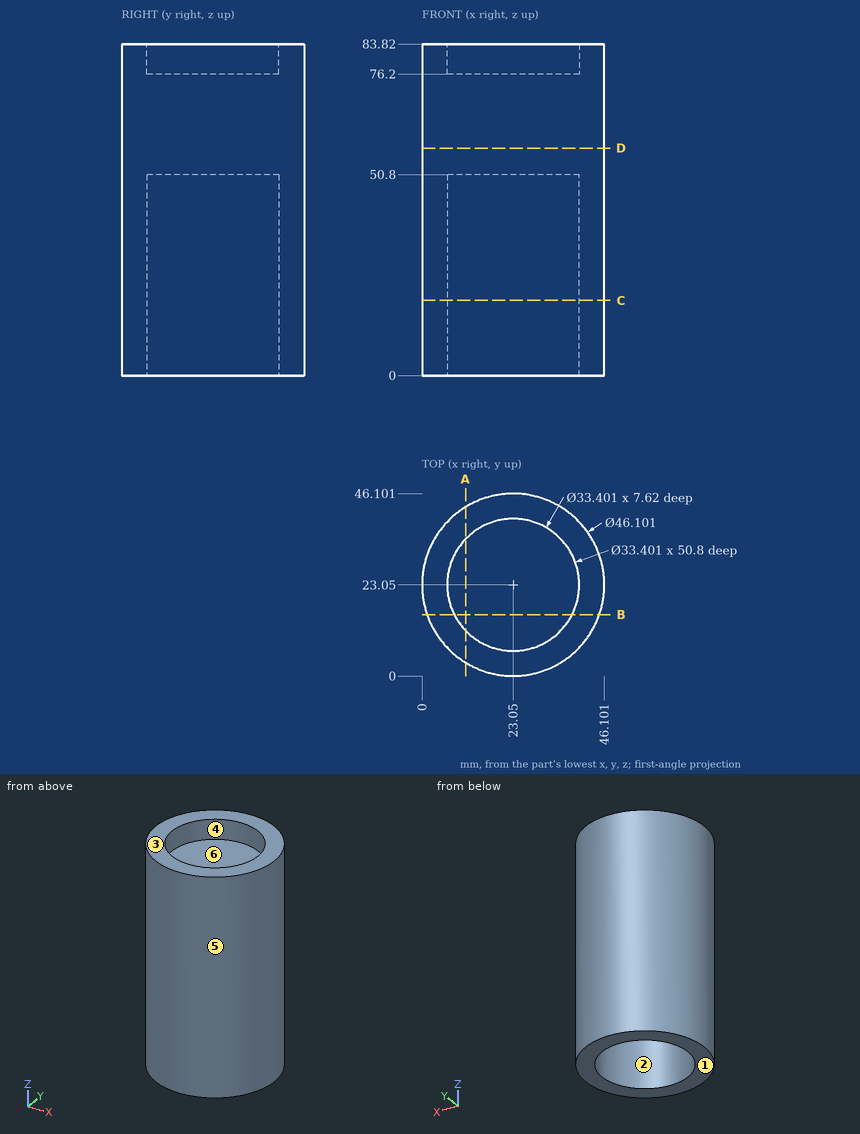
Answer from the drawing. Dimensions are ordinates in mm from the lowest x, y and z of the part. A direction names the side the tool comes from. Coordinates: 2 decimals unless noted, no trailing zeros. Write each loop counter-clockwise with the first axis right and the second up, starting at its lowest first coordinate (ties: lowest second). Pieces come first, ordered by that corner, then holes. Notation, with made-up numbers: M 42,42.25 L 48,42.25 A12 cw 48,62.25 Z; hole C 85.5,22.5 d3. An arc over 180 degrees is marked long. Use one line per item in the form item = value. Start each with the question number.
1. The part is cut by section A-A (x = 11). Give the vertices of the cut face in (y, z), plus the area to 3 significant figures.
2. Straight lines are drawn through the part: probe 1 along Z at (x, y) = (37, 22); probe 2 along Y at (x, z) = (18, 78); probe 3 along X at (y, z) = (15, 22.5). For each, find the intervals that lie inside material, in ascending order. Write a range as from..to.
3. The part is cut by section C-C (z = 19). Give the vertices of the cut face in (x, y).
4. A tool of negligible diameter and unlimited length cuts with its end or side. For the marked faces 1 and 2, from which of +Z, -Z, +X, -X, +Y, -Y can it reach the whole face along a straight path? Write none if from no direction.
5. The part is cut by section D-D (z = 57.5). Give the vertices of the cut face in (x, y), plus the area to 3 significant figures.
6. The mould has two halves that part along Y. Classify the marked faces 3, 4, 5 and 6: released by +Y, released by -Y, zero draft, split by the parting line, or undercut.
7. The part is cut by section B-B (y = 15.5). Give the vertices of the cut face in (x, z) (1 decimal), plus the area to 3 significant figures.
8. Each of these flat-tipped pins is pushed along its axis until it touches: P1, Ø16.5, axis at x = 17, y = 28.5, coming from the +Z side; P2, Ø5, axis at y = 19.5, z = 56, coming from the -X side; P3, Ø6, axis at x = 32, y = 15, coming from the -Z side. Where does it stop, or does it pass through?
Evaluation:
q1.outline = M 3.4,0 L 11.49,0 L 11.49,50.8 L 34.61,50.8 L 34.61,0 L 42.7,0 L 42.7,83.82 L 34.61,83.82 L 34.61,76.2 L 11.49,76.2 L 11.49,83.82 L 3.4,83.82 Z
q1.area = 1,940 mm^2
q2.probe_1 = 50.8..76.2
q2.probe_2 = 0.56..7.13, 38.97..45.54
q2.probe_3 = 1.45..8.42, 37.68..44.65
q3.outline = C 23.05,23.05 d46.1; hole C 23.05,23.05 d33.4
q4.face_1 = -Z, +X, -X, +Y, -Y
q4.face_2 = -Z
q5.outline = C 23.05,23.05 d46.1
q5.area = 1,670 mm^2
q6.face_3 = zero draft
q6.face_4 = undercut
q6.face_5 = split by the parting line
q6.face_6 = undercut
q7.outline = M 1.3,0 L 8.2,0 L 8.2,50.8 L 37.9,50.8 L 37.9,0 L 44.8,0 L 44.8,83.8 L 37.9,83.8 L 37.9,76.2 L 8.2,76.2 L 8.2,83.8 L 1.3,83.8 Z
q7.area = 1,910 mm^2
q8.P1 = 76.2
q8.P2 = 0.02
q8.P3 = 50.8
